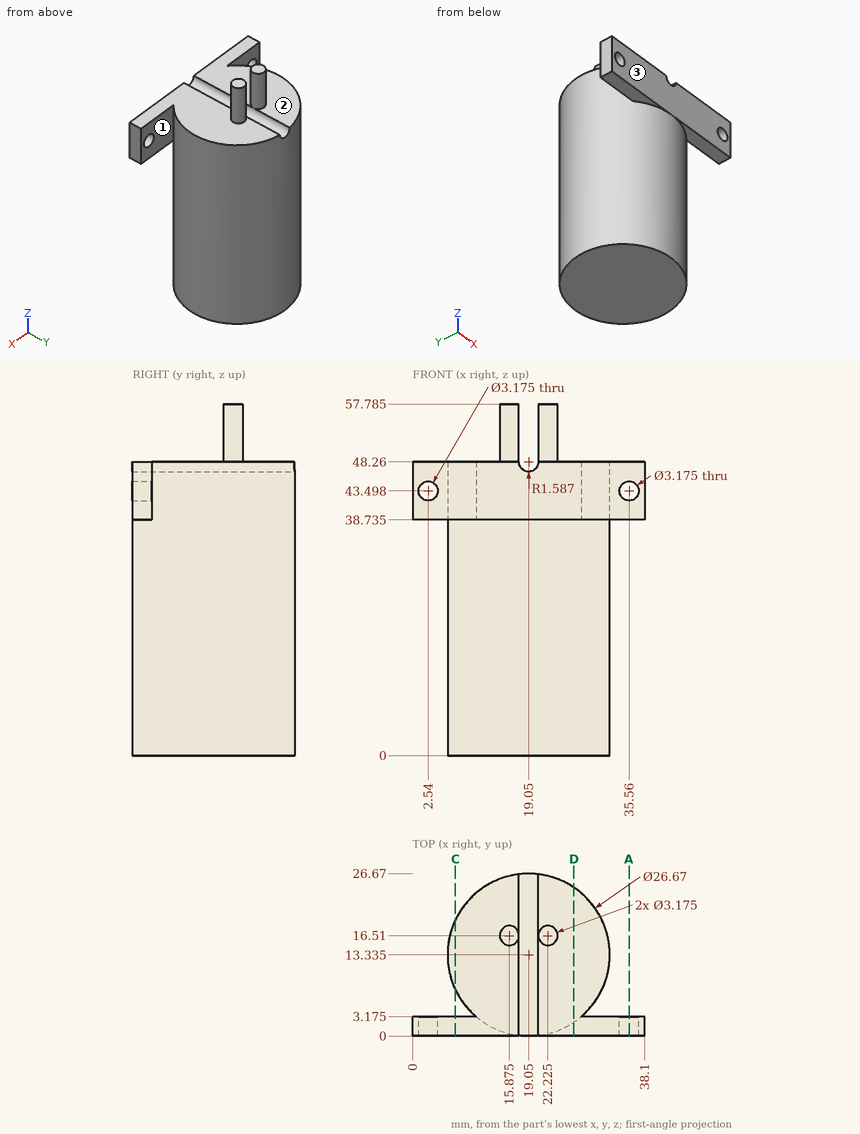
Drawing for the job (mm, zero at the part's lowest x, y, z). Coordinates: 2 decimals unless noted, no trailing zeros. Order: outer loops, then holes, each group sorted by start corner. A loop starts at its lowest first (then second) coordinate and runs counter-clockwise, first axis right, second up.
Item 1: Band-saw the part on D-D on x = 26.5. List the corners of the cut face in (y, z) (1 decimal).
Check sheet entries:
outline: (0, 38.7) - (2.3, 38.7) - (2.3, 0) - (24.4, 0) - (24.4, 48.3) - (0, 48.3) - close
Item 2: Drill centre lines: L1, parallel to Z at x = 35.56, y = 2.1 (1 decimal); L2, parallel to X at y = 21, z = 47.5 (1 decimal); L3, parallel to X at y = 10, z = 48 (1 decimal). Where is each one in solid material? Low to high.
Check sheet entries:
L1: z = 38.7 to 41.9, 45.1 to 48.3
L2: x = 8.1 to 17.7, 20.4 to 30
L3: x = 6.1 to 17.5, 20.6 to 32
Item 3: Pin check, flat tips, straight feed: pin 1 Ø12 at (y, z) = (17, 32) entering from +X (1 decimal); pin 2 Ø1 at (x, y) = (8.5, 2) entering from -Z (1 decimal); pin 3 Ø3 at (x, z) = (3, 42) entering from +Y (1 decimal); pin 4 Ø3 at (x, z) = (2.54, 43.5) entering from -Y. Stop position of each tip, or through.
Check sheet entries:
pin 1: stops at x = 32.4
pin 2: stops at z = 38.7
pin 3: stops at y = 3.2
pin 4: passes through
Item 4: Band-saw the part on C-C on x = 7. List the corners of the cut face in (y, z) (1 decimal).
Check sheet entries:
outline: (0, 38.7) - (3.2, 38.7) - (3.2, 48.3) - (0, 48.3) - close; (7.6, 0) - (19, 0) - (19, 48.3) - (7.6, 48.3) - close
Item 5: Two-plate mould, pull along Y, no slides. Class the marked faces 1, 2 and 3: +Y half, -Y half, draft (parallel to the pull), parting line (faces both ways), or undercut.
Check sheet entries:
face 1: undercut
face 2: draft
face 3: -Y half
Item 6: Band-saw the part on A-A on x = 35.56. List the corners of the cut face in (y, z) (1 decimal).
Check sheet entries:
outline: (0, 38.7) - (3.2, 38.7) - (3.2, 41.9) - (0, 41.9) - close; (0, 45.1) - (3.2, 45.1) - (3.2, 48.3) - (0, 48.3) - close
